```python
from build123d import *

# Parameters (mm, degrees)
F1_DEPTH = 12.7
F3_DEPTH = 12.7
F4_SIZE  = 5.08
F5_T     = -2.54
F6_R     = 5.08
F7_R     = 5.08


with BuildPart() as f1:
    # F0 (on Top) → F1 (new body)
    with BuildSketch(Plane.XY):
        Polygon((-29.5936651047, 42.7012435267), (-20.7587903276, 28.1868066845), (-3.0799934127, 28.5968528045), (4.6840362066, 42.572935257), align=None)
        Polygon((-3.0799934127, 28.5968528045), (6.1145154014, 13.4915886278), (23.8648758049, 13.903294608), (4.6840362066, 42.572935257), align=None)
        Polygon((6.1145154014, 13.4915886278), (-2.3697726995, -2.0237216688), (7.8208672829, -20.1170971814), (23.8648758049, 13.903294608), align=None)
        Polygon((-2.3697726995, -2.0237216688), (-20.0485696143, -2.4337677888), (-25.8524047196, -20.1170971814), (7.8208672829, -20.1170971814), align=None)
        Polygon((-25.8524047196, -20.1170971814), (-20.0485696143, -2.4337677888), (-29.2430784284, 12.6714963879), (-46.4981990716, 12.2712771137), align=None)
        Polygon((-46.4981990716, 12.2712771137), (-29.2430784284, 12.6714963879), (-20.7587903276, 28.1868066845), (-29.5936651047, 42.7012435267), align=None)
        Polygon((-29.2430784284, 12.6714963879), (-20.0485696143, -2.4337677888), (-2.3697726995, -2.0237216688), (6.1145154014, 13.4915886278), (-3.0799934127, 28.5968528045), (-20.7587903276, 28.1868066845), align=None)
    extrude(amount=F1_DEPTH)

    # F2 (on face) → F3 (join)
    with BuildSketch(Plane.XY.offset(12.7)):
        Polygon((-20.9390962878, -2.3024461698), (-2.6609753808, -2.3024461698), (6.4780850727, 13.5268708691), (-2.6609753808, 29.356187908), (-20.9390962878, 29.356187908), (-30.0781567413, 13.5268708691), align=None)
    extrude(amount=F3_DEPTH)

    # F4
    f4_edges = [f1.edges().sort_by_distance(p)[0] for p in [
        (1.908555, 5.612212, 25.4),
        (1.908555, 21.441529, 25.4),
        (-11.800036, 29.356188, 25.4),
        (-25.508627, 21.441529, 25.4),
        (-25.508627, 5.612212, 25.4),
        (-11.800036, -2.302446, 25.4),
    ]]
    chamfer(f4_edges, length=F4_SIZE)

    # F5
    f5_openings = [f1.faces().sort_by_distance(p)[0] for p in [
        (15.842872, -3.106901, 6.35),
        (-9.015769, -20.117097, 6.35),
        (14.274456, 28.238115, 6.35),
        (-12.454814, 42.637089, 6.35),
        (-38.045932, 27.48626, 6.35),
    ]]
    offset(amount=F5_T, openings=f5_openings, kind=Kind.INTERSECTION)

    # F6
    f6_edges = [f1.edges().sort_by_distance(p)[0] for p in [
        (-36.175302, -3.92291, 12.7),
    ]]
    fillet(f6_edges, radius=F6_R)

    # F7
    f7_edges = [f1.edges().sort_by_distance(p)[0] for p in [
        (-36.175302, -3.92291, 0),
    ]]
    fillet(f7_edges, radius=F7_R)


solid = f1.part
```
Can you work these out from the model? Positions are in its coordinate system, mm. A direction names the side the tool comes from. Coordinates: 2 decimals unless noted, no trailing zeros. Loops run counter-clockwise (first coordinate to the right, second up) from the corner with the lowest first, then second, coordinate; pieces in that order, holes last. Notation, with made-up numbers: (19.25, 1.25) -> (46.25, 1.25) arc R18 cw to (46.25, 33.25) -> close; hole circle Ø5 at (58, -9.5). An arc over 180 degrees is marked (long way). Put each result on its own line as item: value. Start each with the question number.
Q1. I want a section at D-D (z = 21.75). Write out the boundary of the cut face in (x, y).
Q2. I'm going to push flat-ended pins straight in: P1, Ø4.5, axis at x = -9, z = 15, coming from the +Y side; P2, Ø1, axis at x = 15, y = -5.5, coming from the +Z side; P3, Ø2, axis at x = 10.5, z = 15.5, coming from the -Y side; P4, Ø6, axis at x = -15.5, z = 17, coming from the -Y side. Where does each tip first touch, or does it pass through?
Q3. I want a section at C-C (y = 25.5). Write out the boundary of the cut face in (x, z), plus the area to 3 significant figures.
Q4. I want a section at A-A (x = -12). Write out the boundary of the cut face in (y, z).
Q5. For faces 1 (the face through (-23.26, 20.26, 14.65)), 2 (the face through (-25.445, 21.552, 16.457)), 3 (the face through (-12, 29.356, 16)), 4 (the face through (-25.57, 5.72, 16.46)), 5 (the face through (14.409, 28.037, 11.412)), which set-ups out of +Z, -Z, +X, -X, +Y, -Y let a thin tool reach every point of the face, with its end or its side?
Q6. I want a section at B-B (z = 14.5). Write out the boundary of the cut face in (x, y).
Q7. Thinking about a two-plate mould opening in Y: for faces 6 (the face through (-12, 14, 22.86)), 7 (the face through (1.845, 5.501, 16.457)), 8 (the face through (-21.79, 7.89, 21.09)), 9 (the face through (-34.12, -2.42, 6.3)), which applies, pulls with the +Y half, pulls with the -Y half, needs draft (parallel to the pull), parting line crosses it, or undercut?
Q8. If I drill on line 1 (Y direction, x = -9.5, z = 17.75); line 2 (Z direction, x = -26, y = -6); line 3 (Y direction, x = 1.5, z = 18.75), over which ranges is the centre line in solid material (lowest first)? Write a range as [from, to].
Taken from the geometry:
1. outline: (-28.43, 13.53) -> (-20.11, -0.87) -> (-3.49, -0.87) -> (4.83, 13.53) -> (-3.49, 27.93) -> (-20.11, 27.93) -> close; hole (-24.28, 13.53) -> (-18.04, 2.72) -> (-5.56, 2.72) -> (0.68, 13.53) -> (-5.56, 24.33) -> (-18.04, 24.33) -> close
2. P1: stops at y = 29.36
2. P2: stops at z = 12.7
2. P3: passes through
2. P4: stops at y = -2.3
3. outline: (-39.15, 0) -> (16.11, 0) -> (16.11, 2.54) -> (-39.15, 2.54) -> close; (-39.15, 10.16) -> (-20.23, 10.16) -> (-20.23, 19.27) -> (-18.71, 20.58) -> (-4.89, 20.58) -> (-3.37, 19.27) -> (-3.37, 10.16) -> (16.11, 10.16) -> (16.11, 12.7) -> (-0.43, 12.7) -> (-0.43, 20.32) -> (-4.89, 24.18) -> (-18.71, 24.18) -> (-23.17, 20.32) -> (-23.17, 12.7) -> (-39.15, 12.7) -> close
3. area: 351 mm2
4. outline: (-20.12, 0) -> (42.64, 0) -> (42.64, 2.54) -> (-20.12, 2.54) -> close; (-20.12, 10.16) -> (0.24, 10.16) -> (0.24, 19.27) -> (3.83, 22.86) -> (23.22, 22.86) -> (26.82, 19.27) -> (26.82, 10.16) -> (42.64, 10.16) -> (42.64, 12.7) -> (29.36, 12.7) -> (29.36, 20.32) -> (24.28, 25.4) -> (2.78, 25.4) -> (-2.3, 20.32) -> (-2.3, 12.7) -> (-20.12, 12.7) -> close
5. face 1: none
5. face 2: +Z, -X, +Y
5. face 3: +Z, +X, -X, +Y
5. face 4: +Z, -X, -Y
5. face 5: +Z, -Z, +X, +Y
6. outline: (-30.08, 13.53) -> (-20.94, -2.3) -> (-2.66, -2.3) -> (6.48, 13.53) -> (-2.66, 29.36) -> (-20.94, 29.36) -> close; hole (-27.15, 13.53) -> (-19.47, 0.24) -> (-4.13, 0.24) -> (3.55, 13.53) -> (-4.13, 26.82) -> (-19.47, 26.82) -> close
7. face 6: undercut
7. face 7: pulls with the -Y half
7. face 8: undercut
7. face 9: pulls with the +Y half
8. line 1: y = [-2.3, 0.24], [26.82, 29.36]
8. line 2: z = [0, 2.54], [10.16, 12.7]
8. line 3: y = [4.9, 9.98], [17.07, 22.15]
